```python
from build123d import *

# Parameters (mm, degrees)
BOX012_W        = 20
BOX012_H        = 2
BOX012_DEPTH    = 5
BOX011_W        = 7
BOX011_H        = 43
BOX011_DEPTH    = 18
BOX010_W        = 5
BOX010_H        = 73
BOX010_DEPTH    = 38
CHAMFER002_SIZE = 3
CHAMFER003_SIZE = 2


with BuildPart() as cube004:
    # Box012 → Box012 (new body)
    with BuildSketch(Plane(origin=(20, -4, 16), x_dir=(1, 0, 0), z_dir=(0, 0, 1))):
        with Locations((10, 1)):
            Rectangle(BOX012_W, BOX012_H)
    extrude(amount=BOX012_DEPTH)


with BuildPart() as obj1:
    # Box011 → Box011 (new body)
    with BuildSketch(Plane(origin=(16, -60, 14), x_dir=(1, 0, 0), z_dir=(0, 0, 1))):
        with Locations((3.5, 21.5)):
            Rectangle(BOX011_W, BOX011_H)
    extrude(amount=BOX011_DEPTH)


with BuildPart() as obj2:
    # Box010 → Box010 (new body)
    with BuildSketch(Plane(origin=(17, -75, 5), x_dir=(1, 0, 0), z_dir=(0, 0, 1))):
        with Locations((2.5, 36.5)):
            Rectangle(BOX010_W, BOX010_H)
    extrude(amount=BOX010_DEPTH)

    # Cut028: cut obj1
    add(obj1.part, mode=Mode.SUBTRACT)

    # Chamfer002
    chamfer002_edges = [obj2.edges().sort_by_distance(p)[0] for p in [
        (17, -38.5, 43),
        (17, -2, 24),
    ]]
    chamfer(chamfer002_edges, length=CHAMFER002_SIZE)

    # Chamfer003
    chamfer003_edges = [obj2.edges().sort_by_distance(p)[0] for p in [
        (17, -38.5, 14),
        (17, -17, 23),
        (17, -38.5, 32),
        (17, -60, 23),
    ]]
    chamfer(chamfer003_edges, length=CHAMFER003_SIZE)

    # Fusion001032: union Cube004
    add(cube004.part)


solid = obj2.part
```
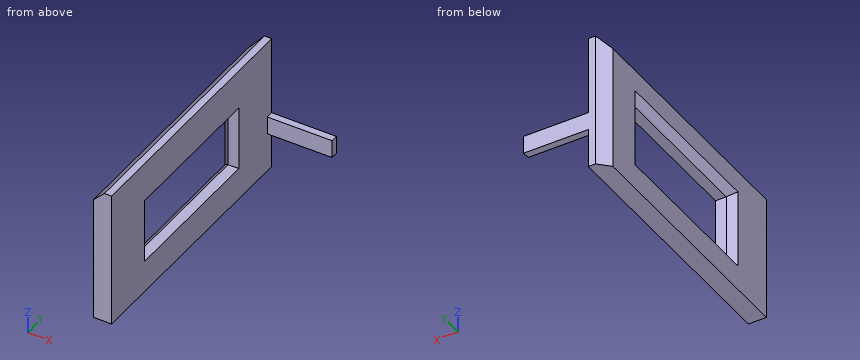
Input: part model. Units: mm. Frame: model coordinates. Round coordinates to 2 decimals unless told otherwise and drop trailing zeros. Loops run counter-clockwise (first coordinate to the right, second up) from the corner with the lowest first, then second, coordinate; pieces in that order, holes last. Notation, with made-up numbers: (18.25, 20) - (31.25, 20) arc R33 cw to (31.25, 48) - close; hole circle Ø6 at (8, -35.5). An arc over 180 degrees is marked (long way). One line per item, written item: value. Start each with the question number.
(1) Contact query for flat-ended pins moving along their axis: P1, Ø2, axis at x = 27, y = -3, coming from the -Z side; P2, Ø12, axis at y = -46.5, z = 18.5, coming from the -X side; P3, Ø8, axis at y = -13.5, z = 30.5, coming from the +X side; P4, Ø8, axis at x = 35.5, z = 15, coming from the +Y side. Output: stop coordinate, or through.
(2) Section A-A, the plane z = 31. Return loops of the section in (x, y), plus the area to 4 significant figures.
(3) Section D-D, the plane z = 19. Return loops of the section in (x, y), plus the area to 4 significant figures.
(4) Section C-C, the plane x = 20.75. Return loops of the section in (y, z), plus the area to 3 significant figures.
(5) Section B-B, the plane y = -37. Return loops of the section in (x, z).
(6) Ray query, line 1 (X direction, y = -67.5, z = 34.5); line 2 (Y direction, x = 19, z = 26); line 3 (Z direction, x = 18, y = -38). Return the intervals inside material, ascending. Write a range as [from, to].
Results below:
1. P1: z = 16
1. P2: x = 17.5
1. P3: x = 22
1. P4: y = -2
2. outline: (17, -75) - (22, -75) - (22, -60) - (19, -60) - (17, -62) - close; (17, -15) - (19, -17) - (22, -17) - (22, -2) - (20, -2) - (17, -5) - close
2. area: 141.5 mm^2
3. outline: (17, -75) - (22, -75) - (22, -60) - (19, -60) - (17, -62) - close; (17, -15) - (19, -17) - (22, -17) - (22, -4) - (40, -4) - (40, -2) - (20, -2) - (17, -5) - close
3. area: 177.5 mm^2
4. outline: (-75, 5) - (-2, 5) - (-2, 43) - (-75, 43) - close; hole (-60, 14) - (-17, 14) - (-17, 32) - (-60, 32) - close
4. area: 2,000 mm^2
5. outline: (17, 5) - (22, 5) - (22, 14) - (19, 14) - (17, 12) - close; (17, 34) - (19, 32) - (22, 32) - (22, 43) - (20, 43) - (17, 40) - close
6. line 1: [17, 22]
6. line 2: [-75, -60], [-17, -3]
6. line 3: [5, 13], [33, 41]
